from build123d import *

# Parameters (mm, degrees)
F2_W     = 85
F2_H     = 130
F3_DEPTH = 4
F4_D     = 3.6
F4_DEPTH = 4
F4_TIP   = 1.0815491142


with BuildPart() as f3:
    # F2 (on Top) → F3 (new body)
    with BuildSketch(Plane.XY):
        Rectangle(F2_W, F2_H)
    extrude(amount=F3_DEPTH)

    # F4
    with Locations(Plane(origin=(0, 0, 0), x_dir=(1, 0, 0), z_dir=(0, 0, -1))):
        with Locations((38.5, -61), (38.5, 61), (-38.5, 61), (-38.5, -61)):
            Hole(F4_D / 2, depth=F4_DEPTH)
            with Locations((0, 0, -(F4_DEPTH + F4_TIP / 2))):  # 118° drill point
                Cone(0, F4_D / 2, F4_TIP, mode=Mode.SUBTRACT)


solid = f3.part
Source: CAD feature listing. Evaluate the final solid. Frame: model axes, mm. Give positions to 0.01 mm unless a question says otherwise; leave off trailing zeros. Write each loop counter-clockwise with the first axis right and the second up, starting at its lowest first coordinate (ties: lowest second). Pieces come first, ordered by that corner, then holes. Notation, with made-up numbers: M 1,0 L 7,0 A18 ccw 7,30 Z; hole C 35.25,42.25 d11. An arc over 180 degrees is marked long. Answer as a JSON object with one key per item and string values.
Q1. Mould query, pull axis Y, two halves, no side actions, for faces 1 (the face through (-1, -65, 2)), 2 (the face through (38.734, 59.215, 2.028)), 3 (the face through (-42.5, -1, 2)). Classes: +Y half, -Y half, draft (parallel to the pull), parting line (faces both ways), or undercut.
Geometry check:
{"face 1": "-Y half", "face 2": "undercut", "face 3": "draft"}
Q2. Cut plane A-A, the plane y = -61. Return the cut outline in (x, z), then the cut area to 3 significant figures.
Geometry check:
{"outline": "M -42.5,0 L -40.3,0 L -40.3,4 L -42.5,4 Z; M -36.7,0 L 36.7,0 L 36.7,4 L -36.7,4 Z; M 40.3,0 L 42.5,0 L 42.5,4 L 40.3,4 Z", "area": "311 mm^2"}
Q3. Cut plane B-B, the plane x = -38.5. Return the cut outline in (y, z).
Geometry check:
{"outline": "M -65,0 L -62.8,0 L -62.8,4 L -65,4 Z; M -59.2,0 L 59.2,0 L 59.2,4 L -59.2,4 Z; M 62.8,0 L 65,0 L 65,4 L 62.8,4 Z"}
Q4. Contact query for a flat-ended pin moving along its axis: P1, Ø3, axis at x = -38.5, y = -61, coming from the -Z side. Output: stop coordinate, or through.
Geometry check:
{"P1": "passes through"}
Q5. Ray query, line 1 along X through (y, z) = (61, 1.65); line 2 along Y through (x, z) = (-38.5, 2.8). Return the intervals inside material, ascending.
Geometry check:
{"line 1": "x = -42.5 to -40.3, -36.7 to 36.7, 40.3 to 42.5", "line 2": "y = -65 to -62.8, -59.2 to 59.2, 62.8 to 65"}
